```python
from build123d import *

# Parameters (mm, degrees)
SKETCH1_R           = 10
BOSS_EXTRUDE1_DEPTH = 30
SKETCH2_R           = 14.5
BOSS_EXTRUDE2_DEPTH = 12.34
SKETCH3_R           = 13
BOSS_EXTRUDE3_DEPTH = 4.2
SKETCH4_R           = 15
BOSS_EXTRUDE4_DEPTH = 19
CUT_EXTRUDE1_DEPTH  = 19
FILLET2_R           = 2


with BuildPart() as part:
    # Sketch1 → Boss-Extrude1 (new body)
    with BuildSketch(Plane(origin=(0, 0, 0), x_dir=(1, 0, 0), z_dir=(0, 1, 0))):
        Circle(SKETCH1_R)
    extrude(amount=BOSS_EXTRUDE1_DEPTH)

    # Sketch2 → Boss-Extrude2 (add)
    with BuildSketch(Plane(origin=(0, 30, 0), x_dir=(1, 0, 0), z_dir=(0, 1, 0))):
        Circle(SKETCH2_R)
    extrude(amount=BOSS_EXTRUDE2_DEPTH)

    # Sketch3 → Boss-Extrude3 (add)
    with BuildSketch(Plane(origin=(0, 42.34, 0), x_dir=(1, 0, 0), z_dir=(0, 1, 0))):
        Circle(SKETCH3_R)
    extrude(amount=BOSS_EXTRUDE3_DEPTH)

    # Sketch4 → Boss-Extrude4 (add)
    with BuildSketch(Plane(origin=(0, 46.54, 0), x_dir=(1, 0, 0), z_dir=(0, 1, 0))):
        Circle(SKETCH4_R)
    extrude(amount=BOSS_EXTRUDE4_DEPTH)

    # Sketch5 → Cut-Extrude1 (cut)
    with BuildSketch(Plane(origin=(0, 65.54, 0), x_dir=(1, 0, 0), z_dir=(0, 1, 0))):
        with BuildLine():
            ThreePointArc((-14.866053103, 2.000116283), (-15, 5.8666e-05), (-14.866068747, -2))
            ThreePointArc((-14.866068747, -2), (-14.037575657, 5.4901e-05), (-14.866053103, 2.000116283))
        make_face()
        with BuildLine():
            ThreePointArc((-2, 14.866068747), (5.4901e-05, 14.037575657), (2.000116283, 14.866053103))
            ThreePointArc((2.000116283, 14.866053103), (5.8666e-05, 15), (-2, 14.866068747))
        make_face()
        with BuildLine():
            ThreePointArc((9.097684458, 11.926111583), (9.92610376, 9.926026117), (11.926182746, 9.097591171))
            ThreePointArc((11.926182746, 9.097591171), (10.606643201, 10.606560235), (9.097684458, 11.926111583))
        make_face()
        with BuildLine():
            ThreePointArc((14.866068747, 2), (14.037575657, -5.4901e-05), (14.866053103, -2.000116283))
            ThreePointArc((14.866053103, -2.000116283), (15, -5.8666e-05), (14.866068747, 2))
        make_face()
        with BuildLine():
            ThreePointArc((11.926111583, -9.097684458), (9.926026117, -9.92610376), (9.097591171, -11.926182746))
            ThreePointArc((9.097591171, -11.926182746), (10.606560235, -10.606643201), (11.926111583, -9.097684458))
        make_face()
        with BuildLine():
            ThreePointArc((2, -14.866068747), (-5.4901e-05, -14.037575657), (-2.000116283, -14.866053103))
            ThreePointArc((-2.000116283, -14.866053103), (-5.8666e-05, -15), (2, -14.866068747))
        make_face()
        with BuildLine():
            ThreePointArc((-9.097684458, -11.926111583), (-9.92610376, -9.926026117), (-11.926182746, -9.097591171))
            ThreePointArc((-11.926182746, -9.097591171), (-10.606643201, -10.606560235), (-9.097684458, -11.926111583))
        make_face()
        with BuildLine():
            ThreePointArc((-11.926111583, 9.097684458), (-9.926026117, 9.92610376), (-9.097591171, 11.926182746))
            ThreePointArc((-9.097591171, 11.926182746), (-10.606560235, 10.606643201), (-11.926111583, 9.097684458))
        make_face()
    extrude(amount=-CUT_EXTRUDE1_DEPTH, mode=Mode.SUBTRACT)

    # Fillet2
    fillet2_edges = [part.edges().sort_by_distance(p)[0] for p in [
        (-5.740197286, 65.54, -13.858215438),
        (5.4901e-05, 65.54, -14.037575657),
        (5.740305685, 65.54, -13.858170537),
        (9.92610376, 65.54, -9.926026117),
        (13.858215438, 65.54, -5.740197286),
        (14.037575657, 65.54, 5.4901e-05),
        (13.858170537, 65.54, 5.740305685),
        (9.926026117, 65.54, 9.92610376),
        (5.740197286, 65.54, 13.858215438),
        (-5.4901e-05, 65.54, 14.037575657),
        (-5.740305685, 65.54, 13.858170537),
        (-9.92610376, 65.54, 9.926026117),
        (-13.858215438, 65.54, 5.740197286),
        (-14.037575657, 65.54, -5.4901e-05),
        (-13.858170537, 65.54, -5.740305685),
        (-9.926026117, 65.54, -9.92610376),
    ]]
    fillet(fillet2_edges, radius=FILLET2_R)


solid = part.part
```
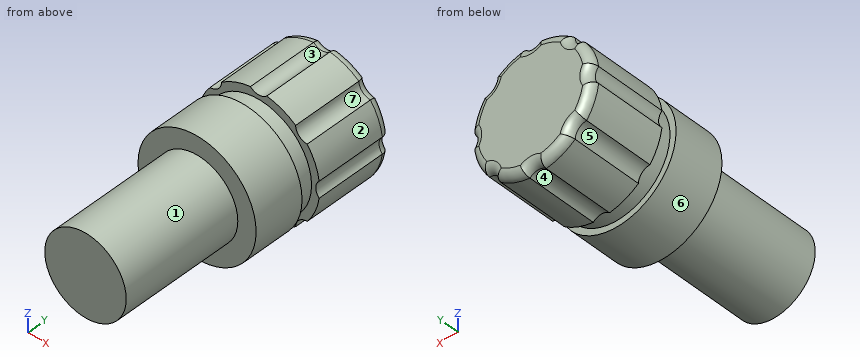
Geometry: final body of the model. Coordinates: model frame, mm. Face numbers are marked on the shaded views. A direction names the side the tool comes from. Round coordinates to 2 decimals unless told otherwise and drop trailing zeros. Write each loop counter-clockwise with the first axis right and the second up, starting at its lowest first coordinate (ties: lowest second). Pieces come first, ordered by that corner, then holes. Notation, with made-up numbers: (48.25, 88) -> (81.25, 88) arc R14 cw to (81.25, 105) -> close; hole circle Ø11 at (48, 78.25). An arc over 180 degrees is marked (long way). Return JSON: item names as keys, results as strings.
Q1. Section A-A on y = 6.5. Return the cut outline in (x, z), and give its area (3 significant figures).
From the geometry:
{"outline": "circle Ø20 at (0, 0)", "area": "314 mm2"}
Q2. Set-up query: the marked faces 4, 5, 6 and 7. Return all of +Z, -Z, +X, -X, +Y, -Y with unobstructed straight access to the full face (end or side cutting, diameter ignored); none if empty.
From the geometry:
{"face 4": "-Z, +Y", "face 5": "-Z, -X, +Y", "face 6": "-Y", "face 7": "+Z, +X, +Y"}
Q3. First-contact query: pin 1 Ø12 at (y, z) = (9.5, 7) entering from -X; pin 2 Ø10 at (y, z) = (9, -3.5) entering from +X; pin 3 Ø6 at (x, y) = (-10, 14.5) entering from +Z. Flat tips, straight axial feed; report the tip coordinate or a pass-through.
From the geometry:
{"pin 1": "x = -9.95", "pin 2": "x = 10", "pin 3": "z = 7.14"}
Q4. Ray query, line 1 (Y direction, x = -7.5, z = 7.25); line 2 (Y direction, x = 3.5, z = 13); line 3 (X direction, y = 29.5, z = 0.5). Return the intervals inside material, ascending.
From the geometry:
{"line 1": "30 to 65.54", "line 2": "30 to 42.34, 46.54 to 65.49", "line 3": "-9.99 to 9.99"}
Q5. Mould query, pull axis X, two halves, no side actions, for the marked faces 1, 2 and 3. Classes: +X half, -X half, draft (parallel to the pull), parting line (faces both ways), or undercut.
From the geometry:
{"face 1": "parting line", "face 2": "+X half", "face 3": "undercut"}
